Geometry check sheet. Reference: the model listing, model coordinates, mm. A direction names the side the tool comes from. Coordinates: 2 decimals unless noted, no trailing zeros. Write each loop counter-clockwise with the first axis right and the second up, starting at its lowest first coordinate (ties: lowest second). Pieces come first, ordered by that corner, then holes. Notation, with made-up numbers: (64.5, -37.75) -> (97.5, -37.75) arc R14 ccw to (97.5, -13.75) -> close; hole circle Ø5 at (-19, 27). An arc over 180 degrees is marked (long way). Answer in a Markdown table with one row per item. Add a question column.
1. Cross-section at B-B on x = 0. Give the number of separate pieces and of enclosed holes in the cut face, and give its area (3 significant figures).
2. Mould release check, pull along Z, two halves, no side actions. Record for faces 4 (the flat face through (0, -22, 16)), 5 (the flat face through (0, 15, 19)), 6 (the cylindrical face through (13.7, -0.06, 17.52)), 7 (the flat face through (0, 22, 16)): pulls with the +Z half, pulls with the -Z half, needs draft (parallel to the pull), parting line crosses it, or undercut.
3. Set-up check for faces 1 (the flat face through (3, -22, 15)), 2 (the flat face through (-22, 0, 13.462)), 3 (the cylindrical face through (0.699, -16.096, 17.521)): record each of +Z, -Z, +X, -X, +Y, -Y from which the full face is reachable in a straight line by a thin tool's end or side.
4. Depth check by flat-ended pin: P1, Ø6.5, axis at x = 1, y = -13.5, coming from the -Z side; P2, Ø12, axis at x = -2.5, z = 8, coming from the -Y side; P3, Ø1, axis at y = 2, z = 6.5, coming from the -X side. Enter the tip coordinate at first touch or a pass-through.
5. Cross-section at A-A on z = 15.25. Record the cut outline in (x, y).
6. Scan lines: L1, parallel to Y at x = -3, z = 6.5; L2, parallel to Z at x = -5.5, y = 13.5; L3, parallel to Z at x = 13, y = 1. Record each from-to range of solid material in increasing order. Write a range as from..to.
7. Cross-section at C-C on z = 3.5. Record the cut outline in (x, y), and give its area (3 significant figures).
```python
from build123d import *

# Parameters (mm, degrees)
SKETCH_R           = 1.3
POCKET_DEPTH       = 1
SKETCH002_W        = 6
SKETCH002_H        = 2.537703
POCKET001_DEPTH    = 3
POLARPATTERN_COUNT = 4
SKETCH003_R        = 3
SKETCH003_R_2      = 1.3
PAD_DEPTH          = 3
CHAMFER_SIZE       = 0.9


with BuildPart() as part:
    # Sketch001 → Revolution (revolve)
    with BuildSketch(Plane.XZ):
        Polygon((0, 20), (19.5, 20), (22.5, 16), (22.5, 0), (21.5, 0), (21.5, 15.999988), (19.249991, 19), (0, 19), align=None)
    revolve(axis=Axis((0, 0, 0), (0, 0, 1)))

    # Sketch (on Face1 of Revolution) → Pocket (cut)
    with BuildSketch(Plane(origin=(0, 0, 20), x_dir=(-1, 0, 0), z_dir=(0, 0, 1))):
        Circle(SKETCH_R)
    extrude(amount=-POCKET_DEPTH, mode=Mode.SUBTRACT)

    # Sketch002 (on DatumPlane) → Pocket001 (cut)
    with BuildSketch(Plane(origin=(0, 22.5, 8), x_dir=(1, 0, 0), z_dir=(0, 1, 0))):
        with Locations((0, -6.731148)):
            Rectangle(SKETCH002_W, SKETCH002_H)
    pocket001 = extrude(amount=-POCKET001_DEPTH, mode=Mode.SUBTRACT)

    # PolarPattern: Pocket001 ×4 about axis
    polarpattern_axis = Axis((0, 0, 0), (0, 0, 1))
    for i in range(1, POLARPATTERN_COUNT):
        add(pocket001.rotate(polarpattern_axis, i * 360 / POLARPATTERN_COUNT), mode=Mode.SUBTRACT)

    # Sketch003 (on Face9 of PolarPattern) → Pad (join)
    with BuildSketch(Plane(origin=(0, 0, 19), x_dir=(1, 0, 0), z_dir=(0, 0, -1))):
        with Locations((-15, 0)):
            Circle(SKETCH003_R)
        with Locations((-15, 0)):
            Circle(SKETCH003_R_2, mode=Mode.SUBTRACT)
        with Locations((0, 15)):
            Circle(SKETCH003_R)
        with Locations((0, 15)):
            Circle(SKETCH003_R_2, mode=Mode.SUBTRACT)
        with Locations((15, 0)):
            Circle(SKETCH003_R)
        with Locations((15, 0)):
            Circle(SKETCH003_R_2, mode=Mode.SUBTRACT)
        with Locations((0, -15)):
            Circle(SKETCH003_R)
        with Locations((0, -15)):
            Circle(SKETCH003_R_2, mode=Mode.SUBTRACT)
    extrude(amount=PAD_DEPTH)

    # Chamfer
    chamfer_edges = [part.edges().sort_by_distance(p)[0] for p in [
        (1.3, 0, 20),
    ]]
    chamfer(chamfer_edges, length=CHAMFER_SIZE)


solid = part.part
```
Results found:
| question | item | result |
|---|---|---|
| 1 | separate pieces | 4 |
| 1 | enclosed holes | 0 |
| 1 | area | 89.7 mm^2 |
| 2 | face 4 | undercut |
| 2 | face 5 | pulls with the -Z half |
| 2 | face 6 | needs draft |
| 2 | face 7 | undercut |
| 3 | face 1 | +Y, -Y |
| 3 | face 2 | +X, -X |
| 3 | face 3 | -Z |
| 4 | P1 | stops at z = 16 |
| 4 | P2 | stops at y = -22.5 |
| 4 | P3 | stops at x = -22.45 |
| 5 | outline | (-22.3, -3) arc R22.5 ccw to (-3, -22.3) -> (-3, -21.29) arc R21.5 cw to (-21.29, -3) -> close; (-22.3, 3) -> (-21.29, 3) arc R21.5 cw to (-3, 21.29) -> (-3, 22.3) arc R22.5 ccw to start; (3, -22.3) arc R22.5 ccw to (22.3, -3) -> (21.29, -3) arc R21.5 cw to (3, -21.29) -> close; (3, 21.29) arc R21.5 cw to (21.29, 3) -> (22.3, 3) arc R22.5 ccw to (3, 22.3) -> close |
| 6 | L1 | y = -22.3..-21.29, 21.29..22.3 |
| 6 | L2 | z = 19..20 |
| 6 | L3 | z = 16..20 |
| 7 | outline | circle Ø45 at (0, 0); hole circle Ø43 at (0, 0) |
| 7 | area | 138 mm^2 |
